For this review, take the finished solid that the model builds, in its own axes (mm). A direction names the side the tool comes from. Give positions to 0.01 mm unless a question says otherwise; leave off trailing zeros. Write each loop counter-clockwise with the first axis right and the second up, starting at its lowest first coordinate (ties: lowest second). Pieces come first, ordered by that corner, then holes. Notation, with made-up numbers: M 14.25,10 L 41.25,10 A29 ccw 41.25,33 Z; hole C 60,10 d7. An arc over 180 degrees is marked long. Use one line per item in the form item = value. Start each with the question number.
Q1. Consider section A-A on y = -1.5. Write out the cut boundary in (x, z).
Q2. Tool access review of faces 1 (the flat face through (-1, -3, -50.5)), 2 (the flat face through (-25, 0, -51)): name each direction out of +Z, -Z, +X, -X, +Y, -Y from which nothing blocks a thin tool from reaching the whole face with its end or side.
Q3. Mouldability with a two-part tool opening along Z and no side actions: class faces 3 (the flat face through (-1, -5, -52.5)), 4 (the flat face through (-1, -9.4, 1)), 5 (the flat face through (-1, -5.4, 1)) as released by +Z, released by -Z, zero draft, split by the parting line, or undercut.
Q4. For probe 1 along Z at (x, y) = (31.5, -1.75); probe 2 along X at (y, z) = (-2.5, -15); probe 3 along Y at (x, z) = (-7.5, 3), list the stretches that pass through material, from the lowest coordinate up. Write a range as [from, to].
Q5. Consider section C-C on x = -13.5. Write out the cut boundary in (y, z), and give its area (3 significant figures).
Q6. Consider section B-B on z = 28. Write out the cut boundary in (x, y), and give its area (3 significant figures).
Q7. Clearance check with a flat-ended pin moving along its axis: pin 1 Ø2 at (x, z) = (34, 30) entering from +Y. State where the tip first meets the part, or that it passes through.
```python
from build123d import *

# Parameters (mm, degrees)
SKETCH1_W           = 110
SKETCH1_H           = 105
SKETCH1_W_2         = 106
SKETCH1_H_2         = 101
BOSS_EXTRUDE1_DEPTH = 5.4
SKETCH2_W           = 110
SKETCH2_H           = 105
BOSS_EXTRUDE2_DEPTH = 4


with BuildPart() as part:
    # Sketch1 → Boss-Extrude1 (new body)
    with BuildSketch(Plane(origin=(0, 0, 0), x_dir=(1, 0, 0), z_dir=(0, 1, 0))):
        Rectangle(SKETCH1_W, SKETCH1_H)
        Rectangle(SKETCH1_W_2, SKETCH1_H_2, mode=Mode.SUBTRACT)
    extrude(amount=-BOSS_EXTRUDE1_DEPTH)

    # Sketch2 → Boss-Extrude2 (add)
    with BuildSketch(Plane.XZ.offset(5.4)):
        Rectangle(SKETCH2_W, SKETCH2_H)
    extrude(amount=BOSS_EXTRUDE2_DEPTH)


solid = part.part
```
Working result:
q1.outline = M -55,-52.5 L 55,-52.5 L 55,52.5 L -55,52.5 Z; hole M -53,-50.5 L 53,-50.5 L 53,50.5 L -53,50.5 Z
q2.face_1 = +Y
q2.face_2 = +Z, -Z, +X, -X, +Y
q3.face_3 = released by -Z
q3.face_4 = zero draft
q3.face_5 = undercut
q4.probe_1 = [-52.5, -50.5], [50.5, 52.5]
q4.probe_2 = [-55, -53], [53, 55]
q4.probe_3 = [-9.4, -5.4]
q5.outline = M -9.4,-52.5 L 0,-52.5 L 0,-50.5 L -5.4,-50.5 L -5.4,50.5 L 0,50.5 L 0,52.5 L -9.4,52.5 Z
q5.area = 442 mm²
q6.outline = M -55,-9.4 L 55,-9.4 L 55,0 L 53,0 L 53,-5.4 L -53,-5.4 L -53,0 L -55,0 Z
q6.area = 462 mm²
q7.pin_1 = -5.4
